Check sheet for the modelled part. Datum: model origin and axes. Units: mm. A direction names the side the tool comes from. Give positions to 0.01 mm unless a question says otherwise; leave off trailing zeros. Write each loop counter-clockwise with the first axis right and the second up, starting at its lowest first coordinate (ties: lowest second). Pieces come first, ordered by that corner, then holes. Notation, with made-up numbers: (37.25, -10) -> (57.25, -10) arc R22 cw to (57.25, 19) -> close; hole circle Ø5 at (9.25, 10.5). An arc over 180 degrees is marked (long way). Answer as a JSON object with one key per item and string values.
from build123d import *

# Parameters (mm, degrees)
BOX_W        = 50
BOX_H        = 40
BOX_DEPTH    = 20
POCKET_DEPTH = 40.001
PAD_DEPTH    = 50


with BuildPart() as pocket:
    # Box → Box (new body)
    with BuildSketch(Plane.XY):
        with Locations((25, 20)):
            Rectangle(BOX_W, BOX_H)
    extrude(amount=BOX_DEPTH)

    # Sketch → Pocket (cut, through all)
    with BuildSketch(Plane.XZ):
        Polygon((12.5, 5), (12.5, 10), (37.5, 10), (37.5, 5), (32.5, 5), (32.5, 0), (17.5, 0), (17.5, 5), align=None)
    extrude(amount=-POCKET_DEPTH, mode=Mode.SUBTRACT)


with BuildPart() as pad:
    # Pad base: copy of Pocket
    add(pocket.part)

    # Sketch001 → Pad (new body)
    with BuildSketch(Plane(origin=(0, 0, 0), x_dir=(0, -1, 0), z_dir=(-1, 0, 0))):
        Polygon((-27.5, 30), (-12.5, 30), (-12.5, 25), (-16, 25), (-16, 10), (-24, 10), (-24, 25), (-27.5, 25), align=None)
    extrude(amount=-PAD_DEPTH)


with BuildPart() as fusion:
    # Fusion base: copy of Pocket
    add(pocket.part)

    # Fusion: union Pad
    add(pad.part)


solid = fusion.part
1. Sectioned sample at A-A, the plane y = 26.5. Enter the section's corners in (x, z), plus the area to 3 significant figures.
Determined:
{"outline": "(0, 0) -> (17.5, 0) -> (17.5, 5) -> (12.5, 5) -> (12.5, 10) -> (37.5, 10) -> (37.5, 5) -> (32.5, 5) -> (32.5, 0) -> (50, 0) -> (50, 20) -> (0, 20) -> close; (0, 25) -> (50, 25) -> (50, 30) -> (0, 30) -> close", "area": "1,050 mm^2"}
2. Sectioned sample at B-B, the plane z = 8. Enter the section's corners in (x, y), plus the area to 3 significant figures.
Determined:
{"outline": "(0, 0) -> (12.5, 0) -> (12.5, 40) -> (0, 40) -> close; (37.5, 0) -> (50, 0) -> (50, 40) -> (37.5, 40) -> close", "area": "1,000 mm^2"}
3. Sectioned sample at C-C, the plane x = 8. Enter the section's corners in (y, z), plus the area to 3 significant figures.
Determined:
{"outline": "(0, 0) -> (40, 0) -> (40, 20) -> (24, 20) -> (24, 25) -> (27.5, 25) -> (27.5, 30) -> (12.5, 30) -> (12.5, 25) -> (16, 25) -> (16, 20) -> (0, 20) -> close", "area": "915 mm^2"}
4. Go/stop test with flat-tipped pins: P1, Ø5.5, axis at x = 31.5, z = 27, coming from the -Y side; P2, Ø1, axis at x = 25, y = 25.5, coming from the -Z side; P3, Ø4, axis at x = 18.5, z = 28.5, coming from the +Y side. Record where each tip stops, or that it passes through.
Determined:
{"P1": "y = 12.5", "P2": "z = 10", "P3": "y = 27.5"}
5. Sectioned sample at D-D, the plane y = 20. Enter the section's corners in (x, z), plus the area to 3 significant figures.
Determined:
{"outline": "(0, 0) -> (17.5, 0) -> (17.5, 5) -> (12.5, 5) -> (12.5, 10) -> (37.5, 10) -> (37.5, 5) -> (32.5, 5) -> (32.5, 0) -> (50, 0) -> (50, 30) -> (0, 30) -> close", "area": "1,300 mm^2"}
6. Access from +Z, -Z, +X, -X, +Y, -Y to the whole of each face (thin tool, end or side, straight path). Record for faces 1 (the face through (32.5, 20, 3)), 2 (the face through (25, 20, 10)), 3 (the face through (25, 8, 20)).
Determined:
{"face 1": "-Z, +Y, -Y", "face 2": "+Y, -Y", "face 3": "+X, -X, -Y"}
7. Scan lines: L1, parallel to Z at x = 13.5, y = 12; L2, parallel to X at y = 12, z = 6.75; L3, parallel to X at y = 23, z = 3. Record each from-to range of solid material in increasing order. Write a range as [from, to].
Determined:
{"L1": "[0, 5], [10, 20]", "L2": "[0, 12.5], [37.5, 50]", "L3": "[0, 17.5], [32.5, 50]"}
